Could you check a few things on this model? Use its own coordinates, in mm. A direction names the side the tool comes from. Coordinates: 2 decimals unless noted, no trailing zeros. Order: outer loops, then holes, each group sorted by start corner. A loop starts at its lowest first (then second) coordinate and runs counter-clockwise, first axis right, second up. Notation, with made-up numbers: M 10,-10.75 L 16,-10.75 A32 ccw 16,20.25 Z; hole C 36,-18 d8. An arc over 180 degrees is marked long. Write item = value, one per line. Start each with the question number.
from build123d import *

# Parameters (mm, degrees)
ESBO_O1_R                = 1.65
RESSALTO_EXTRUS_O1_DEPTH = 2
ESBO_O1_3_W              = 6.3
ESBO_O1_3_H              = 4.6
RESSALTO_EXTRUS_O2_DEPTH = 10
ESBO_O2_W                = 26.421659043
ESBO_O2_H                = 2.598510054
RESSALTO_EXTRUS_O3_DEPTH = 12
RESSALTO_EXTRUS_O4_DEPTH = 2
ESBO_O4_W                = 15.168134441
ESBO_O4_H                = 4.790416537
RESSALTO_EXTRUS_O5_DEPTH = 10
ESBO_O5_W                = 2.278476724
ESBO_O5_H                = 1.465715939
RESSALTO_EXTRUS_O6_DEPTH = 1


with BuildPart() as part:
    # Esboço1 → Ressalto-extrusão1 (new body)
    with BuildSketch(Plane(origin=(0, 0, 0), x_dir=(1, 0, 0), z_dir=(0, 1, 0))):
        Polygon((-49.5, 2), (-30.5, 16.5), (30.5, 16.5), (49.5, 2), (49.5, -16.5), (21, -16.5), (21, -2.5), (-21.3, -2.5), (-21.3, -16.5), (-49.5, -16.5), align=None)
        with Locations((-44.5, 2)):
            Circle(ESBO_O1_R, mode=Mode.SUBTRACT)
        with Locations((44.5, 2)):
            Circle(ESBO_O1_R, mode=Mode.SUBTRACT)
    extrude(amount=RESSALTO_EXTRUS_O1_DEPTH)

    # Esboço1<3> → Ressalto-extrusão2 (add)
    with BuildSketch(Plane(origin=(0, 0, 0), x_dir=(1, 0, 0), z_dir=(0, 1, 0))):
        with Locations((-30.45, -7.45)):
            Rectangle(ESBO_O1_3_W, ESBO_O1_3_H)
        with Locations((-10.8, 10.25)):
            Rectangle(ESBO_O1_3_W, ESBO_O1_3_H)
        with Locations((10.2, 10.25)):
            Rectangle(ESBO_O1_3_W, ESBO_O1_3_H)
        with Locations((30.4, -6.75)):
            Rectangle(ESBO_O1_3_W, ESBO_O1_3_H)
    extrude(amount=-RESSALTO_EXTRUS_O2_DEPTH)

    # Esboço2 → Ressalto-extrusão3 (add)
    with BuildSketch(Plane(origin=(0, 2, 0), x_dir=(1, 0, 0), z_dir=(0, 1, 0))):
        with Locations((-1.359424961, 3.810785195)):
            Rectangle(ESBO_O2_W, ESBO_O2_H)
    extrude(amount=RESSALTO_EXTRUS_O3_DEPTH)

    # Esboço3 → Ressalto-extrusão4 (add)
    with BuildSketch(Plane(origin=(0, 14, 0), x_dir=(1, 0, 0), z_dir=(0, 1, 0))):
        Polygon((-12.779725254, 2.511530168), (10.40079667, 2.511530168), (12.833618236, 4.944351733), (12.833618236, 17.396051346), (11.851404561, 18.378265021), (-12.779725254, 18.378265021), (-14.570254482, 16.587735794), (-14.570254482, 4.107082692), align=None)
    extrude(amount=RESSALTO_EXTRUS_O4_DEPTH)

    # Esboço4 → Ressalto-extrusão5 (add)
    with BuildSketch(Plane(origin=(0, 2, 0), x_dir=(1, 0, 0), z_dir=(0, 1, 0))):
        with Locations((24.193900659, 0.772233303)):
            Rectangle(ESBO_O4_W, ESBO_O4_H)
    extrude(amount=RESSALTO_EXTRUS_O5_DEPTH)

    # Esboço5 → Ressalto-extrusão6 (add)
    with BuildSketch(Plane(origin=(0, 2, 0), x_dir=(1, 0, 0), z_dir=(0, 1, 0))):
        with Locations((-22.531195516, 5.087051721)):
            Rectangle(ESBO_O5_W, ESBO_O5_H)
    extrude(amount=RESSALTO_EXTRUS_O6_DEPTH)


solid = part.part
(1) Imagine slicing it at C-C on x = -44.5. List the corners of the cut face in (y, z) for me, plus the area to 3 significant figures.
(2) Will these pins go through, and if not, where does the flat tip stop? P1, Ø1, axis at x = -34, y = -5, coming from the +Z side; P2, Ø2.5, axis at y = -4.5, z = 7.5, coming from the -X side; P3, Ø5, axis at y = -7, z = 7, coming from the +X side; P4, Ø2, axis at x = 13, y = 12.5, coming from the +Z side.
(3) Thinking about a two-plate mould opening in Y: for faces 1 (the flat face through (-30, -10, 7)), 2 (the flat face through (33.55, -5, 7)), which applies, released by +Y, released by -Y, zero draft, split by the parting line, or undercut?
(4) Please list where these lines run through material, in increasing order: probe 1 along X at (y, z) = (0.6, -2); probe 2 along X at (y, z) = (-2.25, 8.5); probe 3 along Z at (x, y) = (-44.5, 1.2). Write a range as from..to.
(5) Imagine slicing it at A-A on y = -2.5. List the corners of the cut face in (x, z) for me, plus the area to 3 significant figures.
(6) Imagine slicing it at D-D on x = 23.5. List the corners of the cut face in (y, z) for me, plus the area to 3 significant figures.
(7) For faces 3 (the flat face through (-21.3, 1, 9)), 4 (the flat face through (10, -5, -7.95)), 5 (the flat face through (-11, -5, -12.55)), 6 (the flat face through (24, 7, -3.167)), 7 (the flat face through (-7.65, -5, -10)), which set-ups out of +Z, -Z, +X, -X, +Y, -Y let a thin tool reach every point of the face, with its end or its side?
(8) Imagine slicing it at B-B on y = 10.5. List the corners of the cut face in (x, z) for me.
Response:
q1.outline = M 0,-5.82 L 2,-5.82 L 2,-3.65 L 0,-3.65 Z; M 0,-0.35 L 2,-0.35 L 2,16.5 L 0,16.5 Z
q1.area = 38.0 mm2
q2.P1 = 9.75
q2.P2 = -33.6
q2.P3 = 33.55
q2.P4 = through
q3.face_1 = released by -Y
q3.face_2 = zero draft
q4.probe_1 = -49.5..-46.15, -42.85..42.85, 46.15..49.5
q4.probe_2 = -33.6..-27.3, 27.25..33.55
q4.probe_3 = -5.82..-3.65, -0.35..16.5
q5.outline = M -33.6,5.15 L -27.3,5.15 L -27.3,9.75 L -33.6,9.75 Z; M -13.95,-12.55 L -7.65,-12.55 L -7.65,-7.95 L -13.95,-7.95 Z; M 7.05,-12.55 L 13.35,-12.55 L 13.35,-7.95 L 7.05,-7.95 Z; M 27.25,4.45 L 33.55,4.45 L 33.55,9.05 L 27.25,9.05 Z
q5.area = 116 mm2
q6.outline = M 0,-16.5 L 2,-16.5 L 2,-3.17 L 12,-3.17 L 12,1.62 L 2,1.62 L 2,16.5 L 0,16.5 Z
q6.area = 114 mm2
q7.face_3 = +Z, +Y, -Y
q7.face_4 = +Z, +X, -X, -Y
q7.face_5 = -Z, +X, -X, -Y
q7.face_6 = -Z, +X, +Y
q7.face_7 = +Z, -Z, -Y
q8.outline = M -14.57,-5.11 L 11.85,-5.11 L 11.85,-2.51 L -14.57,-2.51 Z; M 16.61,-3.17 L 31.78,-3.17 L 31.78,1.62 L 16.61,1.62 Z
